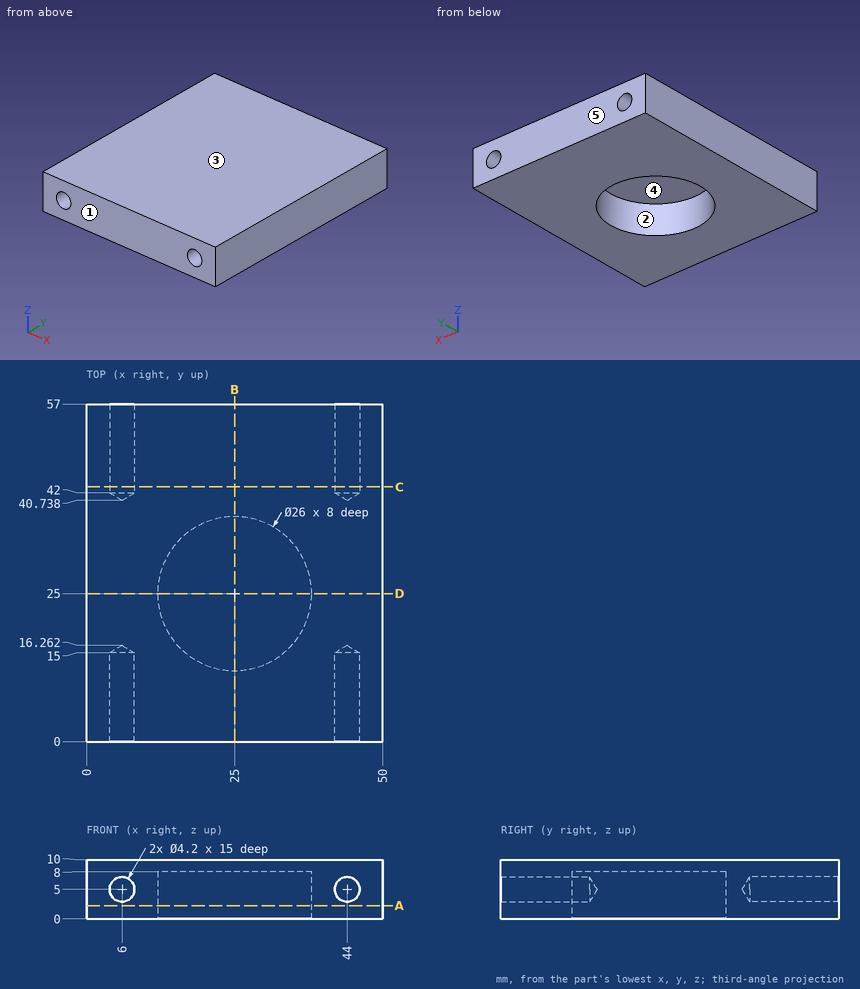
Job drawing, mm, ordinate dimensions from the low corner. One solid piece. A direction names the side the tool comes from. Round coordinates to 2 decimals unless told otherwise and drop trailing zeros. Order: outer loops, then holes, each group sorted by start corner. A loop starts at its lowest first (then second) coordinate and runs counter-clockwise, first axis right, second up. Notation, with made-up numbers: (61.25, 70.25) -> (102.25, 70.25) arc R9 cw to (102.25, 81.25) -> close; hole circle Ø3 at (71.25, 0). An arc over 180 degrees is marked (long way). Answer in a Markdown table with one row per item.
1) Wall check: L1, parallel to Y at x = 25, z = 4.5; L2, parallel to Z at x = 44, y = 48; L3, parallel to Z at x = 19, y = 32. Give the ranges that are in metal, low to high.
Values:
| item | result |
|---|---|
| L1 | 0 to 12, 38 to 57 |
| L2 | 0 to 2.9, 7.1 to 10 |
| L3 | 8 to 10 |
2) Which spindle directions (+Z, -Z, +X, -X, +Y, -Y) get a long thin tool onto all of the face, cutting with end or side? Do the marked faces 1 and 2. Say none if no direction does.
Values:
| item | result |
|---|---|
| face 1 | +Z, -Z, +X, -X, -Y |
| face 2 | -Z |
3) Pin check, flat tips, straight feed: P1, Ø2.5, axis at x = 44, z = 5, coming from the -Y side; P2, Ø3, axis at x = 30, y = 26.5, coming from the -Z side. Stop position of each tip, or through.
Values:
| item | result |
|---|---|
| P1 | y = 15.51 |
| P2 | z = 8 |
4) Band-saw the part on A-A on z = 2.25. Give the cut face in (x, y).
Values:
| item | result |
|---|---|
| outline | (0, 0) -> (50, 0) -> (50, 57) -> (0, 57) -> close; hole circle Ø26 at (25, 25) |
5) Mould opens along Y. For the marked faces 3, 4 and 5 say: released by +Y, released by -Y, zero draft, split by the parting line, or undercut.
Values:
| item | result |
|---|---|
| face 3 | zero draft |
| face 4 | undercut |
| face 5 | released by +Y |
6) Band-saw the part on C-C on y = 43. Give the cut face in (x, z).
Values:
| item | result |
|---|---|
| outline | (0, 0) -> (50, 0) -> (50, 10) -> (0, 10) -> close; hole circle Ø4.2 at (6, 5); hole circle Ø4.2 at (44, 5) |
7) Band-saw the part on D-D on y = 25. Give the cut face in (x, z), and give its area (3 significant figures).
Values:
| item | result |
|---|---|
| outline | (0, 0) -> (12, 0) -> (12, 8) -> (38, 8) -> (38, 0) -> (50, 0) -> (50, 10) -> (0, 10) -> close |
| area | 292 mm2 |
8) Band-saw the part on B-B on x = 25. Give the cut face in (y, z).
Values:
| item | result |
|---|---|
| outline | (0, 0) -> (12, 0) -> (12, 8) -> (38, 8) -> (38, 0) -> (57, 0) -> (57, 10) -> (0, 10) -> close |
